from build123d import *

# Parameters (mm, degrees)
SKETCH1_R                                   = 7.9375
BOSS_EXTRUDE1_DEPTH                         = 4.7625
CSK_FOR_1_4_FLAT_HEAD_MACHINE_SCREW_2_COUNT = 2
CSK_FOR_1_4_FLAT_HEAD_MACHINE_SCREW_2_PITCH = 131.982271537
CSK_FOR_1_4_FLAT_HEAD_MACHINE_SCREW_3_COUNT = 2
CSK_FOR_1_4_FLAT_HEAD_MACHINE_SCREW_3_PITCH = 131.982271537


with BuildPart() as part:
    # Sketch1 → Boss-Extrude1 (new body)
    with BuildSketch(Plane.XY):
        with BuildLine():
            Line((-31.75, 0), (-50.274457233, 62.375531935))
            ThreePointArc((-50.274457233, 62.375531935), (-44.45, 76.989658396), (-28.881566614, 74.726723093))
            Line((-28.881566614, 74.726723093), (15.875, 27.49630657))
            Line((15.875, 27.49630657), (78.9111987, 12.409785423))
            Line((78.9111987, 12.409785423), (130.763159277, 0))
            Line((130.763159277, 0), (79.156023847, -12.351191158))
            Line((79.156023847, -12.351191158), (15.875, -27.49630657))
            Line((15.875, -27.49630657), (-28.881566614, -74.726723093))
            ThreePointArc((-28.881566614, -74.726723093), (-44.45, -76.989658396), (-50.274457233, -62.375531935))
            Line((-50.274457233, -62.375531935), (-31.75, 0))
        make_face()
        Circle(SKETCH1_R, mode=Mode.SUBTRACT)
        with BuildLine():
            Line((9.968214912, 24.497802386), (-25.925542767, 62.375531935))
            ThreePointArc((-25.925542767, 62.375531935), (-31.75, 54.99261314), (-41.056023847, 53.639944611))
            Line((-41.056023847, 53.639944611), (-26.199826659, 3.616173849))
            ThreePointArc((-26.199826659, 3.616173849), (-6.35, 10.998522628), (9.968214912, 24.497802386))
        make_face(mode=Mode.SUBTRACT)
        with BuildLine():
            Line((16.231611747, 20.881628537), (66.981566614, 8.735587325))
            ThreePointArc((66.981566614, 8.735587325), (63.5, 0), (66.981566614, -8.735587325))
            Line((66.981566614, -8.735587325), (16.231611747, -20.881628537))
            ThreePointArc((16.231611747, -20.881628537), (12.7, 0), (16.231611747, 20.881628537))
        make_face(mode=Mode.SUBTRACT)
        with BuildLine():
            Line((88.374457233, 3.615603833), (103.481579639, 0))
            Line((103.481579639, 0), (88.374457233, -3.615603833))
            ThreePointArc((88.374457233, -3.615603833), (88.9, 0), (88.374457233, 3.615603833))
        make_face(mode=Mode.SUBTRACT)
        with BuildLine():
            Line((9.968214912, -24.497802386), (-25.925542767, -62.375531935))
            ThreePointArc((-25.925542767, -62.375531935), (-31.75, -54.99261314), (-41.056023847, -53.639944611))
            Line((-41.056023847, -53.639944611), (-26.199826659, -3.616173849))
            ThreePointArc((-26.199826659, -3.616173849), (-6.35, -10.998522628), (9.968214912, -24.497802386))
        make_face(mode=Mode.SUBTRACT)
    extrude(amount=-BOSS_EXTRUDE1_DEPTH)

    # Sketch3 → CSK for 1/4 Flat Head Machine Screw (100)1 (revolve, cut)
    with BuildSketch(Plane(origin=(76.2, 0, 0), x_dir=(0, -1, 0), z_dir=(1, 0, 0))):
        Polygon((0, 0), (0, 4.7625), (3.3782, 4.7625), (3.3782, 2.568232241), (6.4389, 0), align=None)
    csk_for_1_4_flat_head_machine_screw_100 = revolve(axis=Axis((76.2, 0, 6.35), (0, 0, -1)), mode=Mode.SUBTRACT)

    # CSK for 1_4 Flat Head Machine Screw  2: CSK for 1/4 Flat Head Machine Screw (100)1 ×2
    with Locations(*[Vector(-0.866025404, 0.5, 0) * (i * CSK_FOR_1_4_FLAT_HEAD_MACHINE_SCREW_2_PITCH) for i in range(1, CSK_FOR_1_4_FLAT_HEAD_MACHINE_SCREW_2_COUNT)]):
        add(csk_for_1_4_flat_head_machine_screw_100, mode=Mode.SUBTRACT)

    # CSK for 1_4 Flat Head Machine Screw  3: CSK for 1/4 Flat Head Machine Screw (100)1 ×2
    with Locations(*[Vector(-0.866025404, -0.5, 0) * (i * CSK_FOR_1_4_FLAT_HEAD_MACHINE_SCREW_3_PITCH) for i in range(1, CSK_FOR_1_4_FLAT_HEAD_MACHINE_SCREW_3_COUNT)]):
        add(csk_for_1_4_flat_head_machine_screw_100, mode=Mode.SUBTRACT)


solid = part.part
For this review, take the finished solid that the model builds, in its own axes (mm). A direction names the side the tool comes from. Coordinates: 2 decimals unless noted, no trailing zeros. Order: outer loops, then holes, each group sorted by start corner. A loop starts at its lowest first (then second) coordinate and runs counter-clockwise, first axis right, second up. Notation, with made-up numbers: (16.25, 59.25) - (47.25, 59.25) arc R26 ccw to (47.25, 94.25) - close; hole circle Ø11 at (30.5, 39). An arc over 180 degrees is marked (long way). Answer as CSV lines item,"result". Start each with the question number.
1) To check wall thickness, follow line 1 along Y through (x, z) = (-12.5, -2.25); line 2 along X through (y, z) = (66, -0.9); line 3 along X through (y, z) = (66, -3.6). State the ranges of each line that lie inside material, in increasing order. Write a range as [from, to].
2) Machinability: for faces 5 (the flat face through (41.251, 14.894, -2.348)), 6 (the flat face through (-6.817, 51.442, -2.348)), 7 (the flat face through (-40.883, 30.751, -2.348)), which of the approach directions +Z, -Z, +X, -X, +Y, -Y give a long, thin tool a straight path to every point of the face, cutting with its end or side? Answer none if there is none.
3) Draft analysis for pull direction X (two halves, no side actions). For faces 1 (the cylindrical face through (-38.249, 69.366, -3.65)), 2 (the cylindrical face through (-44.65, 76.87, -2.35)), 3 (the cylindrical face through (12.7, -0.3, -2.3)), 4 (the flat face through (7, 6, 0)), state which applies: +X half, -X half, draft (parallel to the pull), parting line (faces both ways), or undercut.
4) Add section A-A (y = -35.5). State the section outline as (x, z) points, then the cut area to 3 significant figures.
5) Add section B-B (x = -12.5). State the section outline as (y, z) points.
6) Add section C-C (z = -1). Count the separate pieces of the cut face and the enclosed holes in it, then the cut area to 3 significant figures.
7) Add section D-D (x = 76.2). State the section outline as (y, z) points.
8) Insertion check: P1, Ø6, axis at x = -38.1, y = 65.99, coming from the +Z side; P2, Ø1, axis at x = -26, z = -3.5, coming from the +Y side. Each pin has a flat end and moves straight along its axis. Give the tip position at first contact, or say it passes through.
Result:
1,line 1,"[-57.44, -48.21], [-7.88, 7.88], [48.21, 57.44]"
1,line 2,"[-50.8, -43.47], [-32.73, -20.61]"
1,line 3,"[-50.8, -41.48], [-34.72, -20.61]"
2,face 5,"+Z, -Z"
2,face 6,"+Z, -Z, +X, +Y"
2,face 7,"+Z, -Z, -X"
3,face 1,"undercut"
3,face 2,"parting line"
3,face 3,"undercut"
3,face 4,"draft"
4,outline,"(-42.29, -4.76) - (-35.67, -4.76) - (-35.67, 0) - (-42.29, 0) - close; (-0.46, -4.76) - (8.29, -4.76) - (8.29, 0) - (-0.46, 0) - close"
4,area,"73.2 mm^2"
5,outline,"(-57.44, -4.76) - (-48.21, -4.76) - (-48.21, 0) - (-57.44, 0) - close; (-7.88, -4.76) - (7.88, -4.76) - (7.88, 0) - (-7.88, 0) - close; (48.21, -4.76) - (57.44, -4.76) - (57.44, 0) - (48.21, 0) - close"
6,separate pieces,"1"
6,enclosed holes,"8"
6,area,"4,680 mm^2"
7,outline,"(-13.06, -4.76) - (-3.38, -4.76) - (-3.38, -2.57) - (-6.44, 0) - (-13.06, 0) - close; (3.38, -4.76) - (13.06, -4.76) - (13.06, 0) - (6.44, 0) - (3.38, -2.57) - close"
8,P1,"through"
8,P2,"y = 72.21"
